Here's how the part is built. I have some questions about the finished solid (model axes, mm). Face numbers are marked on the shaded views. A direction names the side the tool comes from. Give positions to 0.01 mm unless a question says otherwise; leave off trailing zeros. Write each loop counter-clockwise with the first axis right and the second up, starting at its lowest first coordinate (ties: lowest second). Pieces come first, ordered by that corner, then holes. Notation, with made-up numbers: (50, 35.5) - (57, 35.5) arc R13 cw to (57, 39.5) - close; hole circle Ø6 at (64.5, 58). An arc over 180 degrees is marked (long way). Write each question's results on one line, items separated by ' | '. Start each with the question number.
Item 1: Suppose I cut it at C-C on z = 23. List the corners of the cut face in (x, y) for me (3 decimals).
Item 2: Suppose I cut it at A-A on y = -3.25. List the corners of the cut face in (x, z) for me (1 decimal).
Item 3: Will these pins go through, and if not, where does the flat tip stop? P1, Ø5, axis at y = -2, z = 29.5, coming from the +X side; P2, Ø3, axis at y = -4.5, z = 9, coming from the +X side.
Item 4: Suppose I cut it at B-B on x = 17. List the corners of the cut face in (y, z) for me (3 decimals), then the cut area to 3 significant figures.
Item 5: Which directions (+Z, -Z, +X, -X, +Y, -Y) give clear straight access to the entire face, cutting with the end or side of a thin tool? Please do the marked faces 1 and 2.
Item 6: Please list where these lines run through material, in increasing order: line 1 along Z through (x, y) = (62.5, -0.25); line 2 along X through (y, z) = (-6, 19.5); line 3 along Z through (x, y) = (40.5, -6.5).
```python
from build123d import *

# Parameters (mm, degrees)
F1_DEPTH = 9.525


with BuildPart() as f1:
    # F0 (on Front) → F1 (new body)
    with BuildSketch(Plane.XZ):
        Polygon((62.861793, 62.861793), (0, 0), (9.338706, 0), (38.1, 28.761294), (72.200499, 62.861793), align=None)
        Polygon((9.338706, 0), (0, 0), (0, -9.525), (38.1, -9.525), (38.1, 0), align=None)
        Polygon((38.1, 28.761294), (9.338706, 0), (38.1, 0), align=None)
    extrude(amount=F1_DEPTH)


solid = f1.part
```
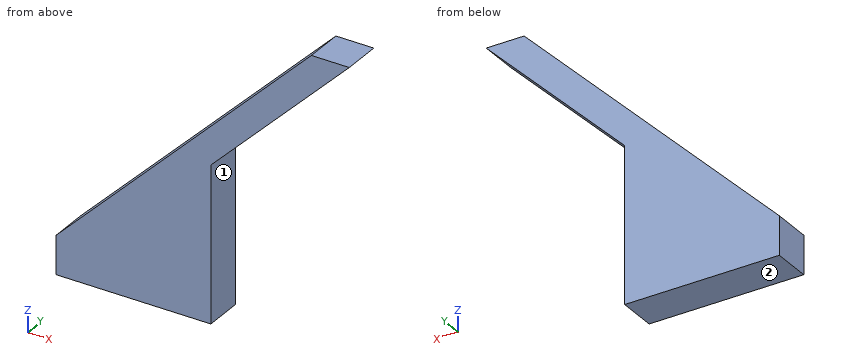
Checked values:
1) outline: (23, -9.525) - (38.1, -9.525) - (38.1, 0) - (23, 0) - close
2) outline: (0, -9.5) - (38.1, -9.5) - (38.1, 28.8) - (72.2, 62.9) - (62.9, 62.9) - (0, 0) - close
3) P1: stops at x = 41.34 | P2: stops at x = 38.1
4) outline: (-9.525, -9.525) - (0, -9.525) - (0, 17) - (-9.525, 17) - close | area: 253 mm^2
5) face 1: -Z, +X, +Y, -Y | face 2: -Z, +X, -X, +Y, -Y
6) line 1: z = 53.16 to 62.5 | line 2: x = 19.5 to 38.1 | line 3: z = 31.16 to 40.5
